```python
from build123d import *

# Parameters (mm, degrees)
F1_DEPTH = 25.4


with BuildPart() as f1:
    # F0 (on Front) → F1 (new body)
    with BuildSketch(Plane.XZ):
        with BuildLine():
            Line((-29.21, 8.636), (-29.21, 0))
            Line((-29.21, 0), (-29.21, -8.636))
            ThreePointArc((-29.21, -8.636), (-28.838026, -9.534026), (-27.94, -9.906))
            Line((-27.94, -9.906), (-8.89, -9.906))
            ThreePointArc((-8.89, -9.906), (-7.991974, -9.534026), (-7.62, -8.636))
            Line((-7.62, -8.636), (-7.62, -5.334))
            ThreePointArc((-7.62, -5.334), (-7.32242, -4.61558), (-6.604, -4.318))
            Line((-6.604, -4.318), (-6.604, -8.128))
            Line((-6.604, -8.128), (0, -8.128))
            Line((0, -8.128), (6.604, -8.128))
            Line((6.604, -8.128), (6.604, -4.318))
            ThreePointArc((6.604, -4.318), (7.32242, -4.61558), (7.62, -5.334))
            Line((7.62, -5.334), (7.62, -8.636))
            ThreePointArc((7.62, -8.636), (7.991974, -9.534026), (8.89, -9.906))
            Line((8.89, -9.906), (27.94, -9.906))
            ThreePointArc((27.94, -9.906), (28.838026, -9.534026), (29.21, -8.636))
            Line((29.21, -8.636), (29.21, 0))
            Line((29.21, 0), (29.21, 8.636))
            ThreePointArc((29.21, 8.636), (28.838026, 9.534026), (27.94, 9.906))
            Line((27.94, 9.906), (8.89, 9.906))
            ThreePointArc((8.89, 9.906), (7.991974, 9.534026), (7.62, 8.636))
            Line((7.62, 8.636), (7.62, 5.334))
            ThreePointArc((7.62, 5.334), (7.32242, 4.61558), (6.604, 4.318))
            Line((6.604, 4.318), (6.604, 8.128))
            Line((6.604, 8.128), (0, 8.128))
            Line((0, 8.128), (-6.604, 8.128))
            Line((-6.604, 8.128), (-6.604, 4.318))
            ThreePointArc((-6.604, 4.318), (-7.32242, 4.61558), (-7.62, 5.334))
            Line((-7.62, 5.334), (-7.62, 8.636))
            ThreePointArc((-7.62, 8.636), (-7.991974, 9.534026), (-8.89, 9.906))
            Line((-8.89, 9.906), (-27.94, 9.906))
            ThreePointArc((-27.94, 9.906), (-28.838026, 9.534026), (-29.21, 8.636))
        make_face()
    extrude(amount=F1_DEPTH)


solid = f1.part
```
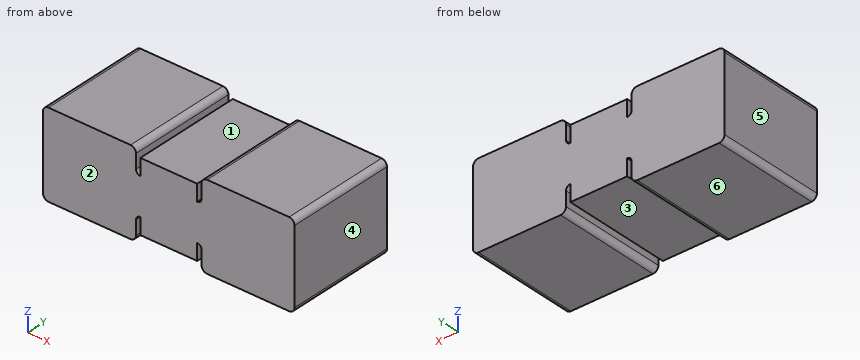
Can you work these out from the model? Positions are in its coordinate system, mm. Face numbers are marked on the shaded views. A direction names the side the tool comes from. Coordinates: 2 decimals unless noted, no trailing zeros. Loops run counter-clockwise (first coordinate to the right, second up) from the corner with the lowest first, then second, coordinate; pieces in that order, holes last. Notation, with made-up numbers: (-21.5, 61) -> (-9.5, 61) arc R22 cw to (-9.5, 89) -> close; hole circle Ø11 at (-1, 31.25). An arc over 180 degrees is marked (long way). Answer as a JSON object with one key per item and string values.
1) Thinking about a two-plate mould opening in X: for the marked faces 3, 4, 5 and 6, which applies, pulls with the +X half, pulls with the -X half, needs draft (parallel to the pull), parting line crosses it, or undercut?
Results:
{"face 3": "undercut", "face 4": "pulls with the +X half", "face 5": "pulls with the -X half", "face 6": "needs draft"}
2) Imagine slicing it at B-B (y = -12). Please give me the cut outline in (x, z).
Results:
{"outline": "(-29.21, -8.64) arc R1.27 ccw to (-27.94, -9.91) -> (-8.89, -9.91) arc R1.27 ccw to (-7.62, -8.64) -> (-7.62, -5.33) arc R1.02 cw to (-6.6, -4.32) -> (-6.6, -8.13) -> (6.6, -8.13) -> (6.6, -4.32) arc R1.02 cw to (7.62, -5.33) -> (7.62, -8.64) arc R1.27 ccw to (8.89, -9.91) -> (27.94, -9.91) arc R1.27 ccw to (29.21, -8.64) -> (29.21, 8.64) arc R1.27 ccw to (27.94, 9.91) -> (8.89, 9.91) arc R1.27 ccw to (7.62, 8.64) -> (7.62, 5.33) arc R1.02 cw to (6.6, 4.32) -> (6.6, 8.13) -> (-6.6, 8.13) -> (-6.6, 4.32) arc R1.02 cw to (-7.62, 5.33) -> (-7.62, 8.64) arc R1.27 ccw to (-8.89, 9.91) -> (-27.94, 9.91) arc R1.27 ccw to (-29.21, 8.64) -> close"}
3) For the marked faces 1 and 2, which set-ups out of +Z, -Z, +X, -X, +Y, -Y let a thin tool reach every point of the face, with its end or its side?
Results:
{"face 1": "+Z, +Y, -Y", "face 2": "+Z, -Z, +X, -X, -Y"}
4) Imagine slicing it at C-C (x = -2). Please give me the cut outline in (y, z).
Results:
{"outline": "(-25.4, -8.13) -> (0, -8.13) -> (0, 8.13) -> (-25.4, 8.13) -> close"}
5) Imagine slicing it at A-A (z = -7.5). Please give me the cut outline in (x, y).
Results:
{"outline": "(-29.21, -25.4) -> (-7.62, -25.4) -> (-7.62, 0) -> (-29.21, 0) -> close; (-6.6, -25.4) -> (6.6, -25.4) -> (6.6, 0) -> (-6.6, 0) -> close; (7.62, -25.4) -> (29.21, -25.4) -> (29.21, 0) -> (7.62, 0) -> close"}
6) For P1, Ø10.5, axis at x = 1, y = -12.5, coming from the +Z side; P2, Ø4, axis at x = 2.5, y = -8.5, coming from the -Z side, each with a flat end and sliding along its axis, tell me the tip position at first contact or that it passes through.
Results:
{"P1": "stops at z = 8.13", "P2": "stops at z = -8.13"}
7) If I drill on line 1 (X direction, y = -2.75, z = 7); line 2 (X direction, y = -18.25, z = 8.5); line 3 (X direction, y = -11, z = -4.75), over which ranges is the centre line in solid material (lowest first)?
Results:
{"line 1": "x = -29.21 to -7.62, -6.6 to 6.6, 7.62 to 29.21", "line 2": "x = -29.21 to -7.62, 7.62 to 29.21", "line 3": "x = -29.21 to -7.44, -6.6 to 6.6, 7.44 to 29.21"}
